Source: CAD feature listing. Evaluate the final solid. Frame: model axes, mm. Give positions to 0.01 mm unless a question says otherwise; leave off trailing zeros. Write each loop counter-clockwise with the first axis right and the second up, starting at its lowest first coordinate (ties: lowest second). Pieces come first, ordered by that corner, then holes. Notation, with made-up numbers: M 52.5,-28 L 57.5,-28 A18 ccw 57.5,-21 Z; hole C 32,59.25 d4. An arc over 180 degrees is marked long. Return JSON: item names as keys, results as strings.
```python
from build123d import *

# Parameters (mm, degrees)
BOSS_EXTRUDE1_DEPTH      = 750
BOSS_EXTRUDE1_DEPTH_BACK = 750
SKETCH3_R                = 6
CHAMFER1_SIZE            = 0.24
SKETCH5_R                = 0.04114626
CUT_EXTRUDE2_DEPTH       = 751.047998464


with BuildPart() as part:
    # Sketch3 → Boss-Extrude1 (new, two sides: drawn at the far end of the back side and taken through both)
    with BuildSketch(Plane.XY.offset(-BOSS_EXTRUDE1_DEPTH_BACK)):
        Circle(SKETCH3_R)
    extrude(amount=BOSS_EXTRUDE1_DEPTH + BOSS_EXTRUDE1_DEPTH_BACK)

    # Chamfer1
    chamfer1_edges = [part.edges().sort_by_distance(p)[0] for p in [
        (-6, 0, -750),
        (-6, 0, 750),
    ]]
    chamfer(chamfer1_edges, length=CHAMFER1_SIZE)

    # Sketch5 → Cut-Extrude2 (cut, through all)
    with BuildSketch(Plane(origin=(0, 0, 0), x_dir=(1, 0, 0), z_dir=(0, 1, 0))):
        with Locations(Location((0, 0, 0), (0, 0, 270))):
            Circle(SKETCH5_R)
    extrude(amount=-CUT_EXTRUDE2_DEPTH, mode=Mode.SUBTRACT)


solid = part.part
```
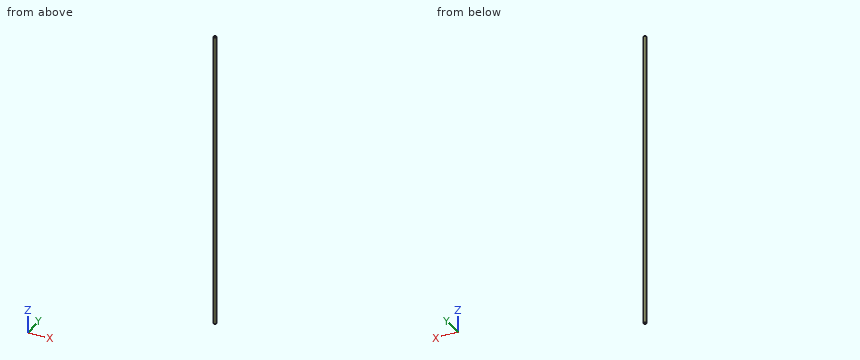
1) Contact query for flat-ended pins moving along their axis: pin 1 Ø4 at (y, z) = (-3.5, 547) entering from -X; pin 2 Ø1 at (y, z) = (4.5, -202) entering from +X; pin 3 Ø3 at (y, z) = (-2.5, -168.5) entering from +X. Output: stop coordinate, or through.
Numbers:
{"pin 1": "stops at x = -5.81", "pin 2": "stops at x = 4.47", "pin 3": "stops at x = 5.92"}
2) Cut plane A-A, the plane z = -72. Return the cut outline in (x, y), then the cut area to 3 significant figures.
Numbers:
{"outline": "C 0,0 d12", "area": "113 mm²"}
3) Line query: line 1 (Y direction, x = 1.75, z = 635.5); line 2 (Y direction, x = 1, z = -654.5); line 3 (X direction, y = 0.75, z = 429). Output: solid intervals per line, ascending. Write a range as [from, to].
Numbers:
{"line 1": "y = [-5.74, 5.74]", "line 2": "y = [-5.92, 5.92]", "line 3": "x = [-5.95, 5.95]"}
